The listing builds one solid part. Answer for the finished solid, in the listing's coordinates (mm). A direction names the side the tool comes from. Give positions to 0.01 mm unless a question says otherwise; leave off trailing zeros. Write each loop counter-clockwise with the first axis right and the second up, starting at its lowest first coordinate (ties: lowest second). Pieces come first, ordered by that corner, then holes. Notation, with made-up numbers: (-30, -30.5) - (-6, -30.5) arc R30 ccw to (-6, -1.5) - close; hole circle Ø8 at (37.25, -24.75). An arc over 180 degrees is marked (long way). Return JSON: item names as keys, results as strings.
from build123d import *

# Parameters (mm, degrees)
BOSS_EXTRUDE1_DEPTH = 25.4
BOSS_EXTRUDE2_DEPTH = 25.4
CUT_EXTRUDE1_DEPTH  = 51.8


with BuildPart() as part:
    # Sketch1 → Boss-Extrude1 (new body)
    with BuildSketch(Plane(origin=(0, 0, 0), x_dir=(1, 0, 0), z_dir=(0, 1, 0))):
        with BuildLine():
            ThreePointArc((3.812810865, 2.209805629), (4.255786873, 1.144135352), (4.4069, 0))
            ThreePointArc((4.4069, 0), (-1.144135352, -4.255786873), (-3.812810865, 2.209805629))
            ThreePointArc((-3.812810865, 2.209805629), (-4.50575261, 4.813242153), (-7.109189135, 4.120300408))
            ThreePointArc((-7.109189135, 4.120300408), (-2.133301363, -7.935141518), (8.2169, 0))
            ThreePointArc((8.2169, 0), (7.935141518, 2.133301363), (7.109189135, 4.120300408))
            ThreePointArc((7.109189135, 4.120300408), (4.50575261, 4.813242153), (3.812810865, 2.209805629))
        make_face()
    extrude(amount=BOSS_EXTRUDE1_DEPTH)

    # Sketch2 → Boss-Extrude2 (add)
    with BuildSketch(Plane(origin=(0, 25.4, 0), x_dir=(1, 0, 0), z_dir=(0, 1, 0))):
        with BuildLine():
            ThreePointArc((-7.109189135, 4.120300408), (0, -8.2169), (7.109189135, 4.120300408))
            ThreePointArc((7.109189135, 4.120300408), (4.50575261, 4.813242153), (3.812810865, 2.209805629))
            ThreePointArc((3.812810865, 2.209805629), (0, -4.4069), (-3.812810865, 2.209805629))
            ThreePointArc((-3.812810865, 2.209805629), (-4.50575261, 4.813242153), (-7.109189135, 4.120300408))
        make_face()
        with BuildLine():
            ThreePointArc((2.52722334, 1.464712665), (2.820838561, 0.758360608), (2.921, 0))
            ThreePointArc((2.921, 0), (-0.758360608, -2.820838561), (-2.52722334, 1.464712665))
            ThreePointArc((-2.52722334, 1.464712665), (-3.490412365, 5.083489434), (-7.109189135, 4.120300408))
            ThreePointArc((-7.109189135, 4.120300408), (-4.50575261, 4.813242153), (-3.812810865, 2.209805629))
            ThreePointArc((-3.812810865, 2.209805629), (0, -4.4069), (3.812810865, 2.209805629))
            ThreePointArc((3.812810865, 2.209805629), (4.50575261, 4.813242153), (7.109189135, 4.120300408))
            ThreePointArc((7.109189135, 4.120300408), (3.490412365, 5.083489434), (2.52722334, 1.464712665))
        make_face()
    extrude(amount=BOSS_EXTRUDE2_DEPTH)

    # Sketch3 → Cut-Extrude1 (cut, through all)
    with BuildSketch(Plane(origin=(0, 50.8, 0), x_dir=(1, 0, 0), z_dir=(0, 1, 0))):
        with BuildLine():
            Line((3.074580558, -7.62), (-3.074580558, -7.62))
            ThreePointArc((-3.074580558, -7.62), (0, -8.2169), (3.074580558, -7.62))
        make_face()
    extrude(amount=-CUT_EXTRUDE1_DEPTH, mode=Mode.SUBTRACT)


solid = part.part
Item 1: A cutting plane is placed at B-B on z = 0.75. Determine the outline of the cut face in (x, y).
Answer below:
{"outline": "(-8.18, 0) - (-4.34, 0) - (-4.34, 25.4) - (-2.82, 25.4) - (-2.82, 50.8) - (-8.18, 50.8) - close; (2.82, 25.4) - (4.34, 25.4) - (4.34, 0) - (8.18, 0) - (8.18, 50.8) - (2.82, 50.8) - close"}
Item 2: A cutting plane is placed at D-D on x = 5.5. Determine the outline of the cut face in (y, z), then the cut area to 3 significant figures.
Answer below:
{"outline": "(0, -5.07) - (25.4, -5.07) - (25.4, -5.35) - (50.8, -5.35) - (50.8, 6.1) - (0, 6.1) - close", "area": "575 mm²"}
Item 3: For faces 4 (the face through (-4, 0, 3)), 5 (the face through (-4.47, 12.52, -4.79)), determine the directions among +Z, -Z, +X, -X, +Y, -Y from which every point of the face is accessible in a straight line to the end or side of a thin tool.
Answer below:
{"face 4": "+Z, -Z, +X, -X, -Y", "face 5": "-Y"}
Item 4: Flat-ended cylindrical pins translate along their axes: P1, Ø6, axis at y = 23.5, z = 5, coming from the +X side; P2, Ø5, axis at y = 8, z = 5, coming from the -X side; P3, Ø1.5, axis at x = 4.5, y = 41, coming from the +Z side. Find the tip coordinate at first contact, or state that the pin passes through.
Answer below:
{"P1": "stops at x = 7.97", "P2": "stops at x = -7.83", "P3": "stops at z = 7.31"}
Item 5: Consider L1, parallel to X at y = 8.5, z = -0.5; L2, parallel to X at y = 25.5, z = -4; L3, parallel to Y at x = 3.75, z = -5. Determine where each line is inside the solid, lowest interval first.
Answer below:
{"L1": "x = -8.2 to -4.38, 4.38 to 8.2", "L2": "x = -7.18 to -2.46, 2.46 to 7.18", "L3": "y = 25.4 to 50.8"}
Item 6: A cutting plane is placed at A-A on x = 0. Determine the outline of the cut face in (y, z).
Answer below:
{"outline": "(0, 4.41) - (25.4, 4.41) - (25.4, 2.92) - (50.8, 2.92) - (50.8, 7.62) - (0, 7.62) - close"}
Item 7: The mould has two halves that part along Z. Classify faces 1 (the face through (-1.94, 50.8, 2.45)), 2 (the face through (0, 26, 7.62)), 3 (the face through (-3, 25.4, -1)): +Z half, -Z half, draft (parallel to the pull), parting line (faces both ways), or undercut.
Answer below:
{"face 1": "draft", "face 2": "+Z half", "face 3": "undercut"}
Item 8: A cutting plane is placed at C-C on y = 18. Determine the outline of the cut face in (x, z) (3 decimals), then the cut area to 3 significant figures.
Answer below:
{"outline": "(-7.109, -4.12) arc R1.905 ccw to (-3.813, -2.21) arc R4.407 cw (long way) to (3.813, -2.21) arc R1.905 ccw to (7.109, -4.12) arc R8.217 ccw to (3.075, 7.62) - (-3.075, 7.62) arc R8.217 ccw to start", "area": "110 mm²"}
